Verification items for the finished model (mm, model axes). Face numbers are marked on the shaded views. A direction names the side the tool comes from. Round coordinates to 2 decimals unless told otherwise and drop trailing zeros. Order: outer loops, then holes, each group sorted by start corner. A loop starts at its lowest first (then second) coordinate and runs counter-clockwise, first axis right, second up. Notation, with made-up numbers: (-37.75, 41.5) -> (6.25, 41.5) arc R12 ccw to (6.25, 46.5) -> close; hole circle Ø6 at (-17, 21.25). An arc over 180 degrees is marked (long way). Return JSON: item names as keys, results as strings. Group by question number.
Item 1: Access from +Z, -Z, +X, -X, +Y, -Y to the whole of each face (thin tool, end or side, straight path). Record for the marked faces 1, 2 and 3.
Item 2: Sectioned sample at D-D on z = 1.75. Record the cut outline in (x, y).
Item 3: Sectioned sample at B-B on x = 5. Record the cut outline in (y, z), plus the area to 3 significant figures.
Item 4: Sectioned sample at A-A on y = -10. Record the cut outline in (x, z), plus the area to 3 significant figures.
Item 5: Sectioned sample at C-C on x = 1.25. Record the cut outline in (y, z), plus the area to 3 significant figures.
Item 6: Scan lines: probe 1 along Y at (x, z) = (5, -8.95); probe 2 along Y at (x, z) = (5, 1.6); probe 3 along Y at (x, z) = (4.25, -2). Record each from-to range of solid material in increasing order. Write a range as from..to.
Item 7: Depth check by flat-ended pin: pin 1 Ø3.5 at (x, y) = (5, -10) entering from +Z; pin 2 Ø3 at (x, z) = (7, -3.5) entering from -Y; pin 3 Ø3 at (x, z) = (3, -5) entering from +Y. Enter the tip coordinate at first touch or a pass-through.
Item 8: Draft check along Y on the marked faces 4, 5, 6 and 7. Enter one of: pulls with the +Y half, pulls with the -Y half, needs draft (parallel to the pull), parting line crosses it, or undercut.
```python
from build123d import *

# Parameters (mm, degrees)
SKETCH1_W           = 10
SKETCH1_H           = 15
SKETCH1_R           = 3
SKETCH1_H_2         = 3
BOSS_EXTRUDE1_DEPTH = 3
SKETCH1_4_W         = 10
SKETCH1_4_H         = 3
BOSS_EXTRUDE2_DEPTH = 10
BOSS_EXTRUDE3_START = -10
SKETCH1_5_W         = 10
SKETCH1_5_H         = 10
SKETCH1_5_R         = 3
BOSS_EXTRUDE3_DEPTH = 3


with BuildPart() as part:
    # Sketch1 → Boss-Extrude1 (new body)
    # profile 1 of 2: a face of its own
    with BuildSketch(Plane.XY):
        with Locations((5, -7.5)):
            Rectangle(SKETCH1_W, SKETCH1_H)
        with Locations((5, -10)):
            Circle(SKETCH1_R, mode=Mode.SUBTRACT)
    # profile 2 of 2: a face of its own
    with BuildSketch(Plane.XY):
        with Locations((5, 1.5)):
            Rectangle(SKETCH1_W, SKETCH1_H_2)
    extrude(amount=BOSS_EXTRUDE1_DEPTH)

    # Sketch1<4> → Boss-Extrude2 (add)
    with BuildSketch(Plane.XY):
        with Locations((5, 1.5)):
            Rectangle(SKETCH1_4_W, SKETCH1_4_H)
    extrude(amount=-BOSS_EXTRUDE2_DEPTH)

    # Sketch1<5> → Boss-Extrude3 (add)
    with BuildSketch(Plane.XY.offset(BOSS_EXTRUDE3_START)):
        with Locations((5, 8)):
            Rectangle(SKETCH1_5_W, SKETCH1_5_H)
        with Locations((5, 8)):
            Circle(SKETCH1_5_R, mode=Mode.SUBTRACT)
    extrude(amount=BOSS_EXTRUDE3_DEPTH)


solid = part.part
```
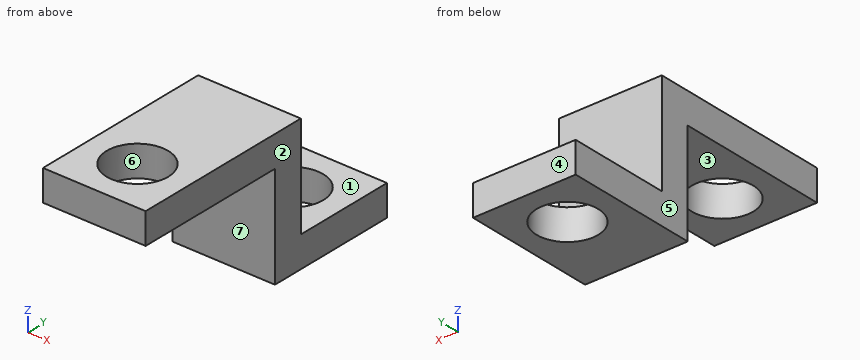
Recorded:
{
 "1": {"face 1": "+Z, +X, -X, +Y", "face 2": "+Z, -Z, +X, +Y, -Y", "face 3": "-Z, +X, -X, -Y"},
 "2": {"outline": "(0, -15) -> (10, -15) -> (10, 3) -> (0, 3) -> close; hole circle Ø6 at (5, -10)"},
 "3": {"outline": "(-15, 0) -> (-13, 0) -> (-13, 3) -> (-15, 3) -> close; (-7, 0) -> (0, 0) -> (0, -10) -> (5, -10) -> (5, -7) -> (3, -7) -> (3, 3) -> (-7, 3) -> close; (11, -10) -> (13, -10) -> (13, -7) -> (11, -7) -> close", "area": "78.0 mm²"},
 "4": {"outline": "(0, 0) -> (2, 0) -> (2, 3) -> (0, 3) -> close; (8, 0) -> (10, 0) -> (10, 3) -> (8, 3) -> close", "area": "12.0 mm²"},
 "5": {"outline": "(-15, 0) -> (0, 0) -> (0, -10) -> (13, -10) -> (13, -7) -> (3, -7) -> (3, 3) -> (-15, 3) -> close", "area": "114 mm²"},
 "6": {"probe 1": "0..5, 11..13", "probe 2": "-15..-13, -7..3", "probe 3": "0..3"},
 "7": {"pin 1": "through", "pin 2": "y = 0", "pin 3": "y = 3"},
 "8": {"face 4": "pulls with the +Y half", "face 5": "needs draft", "face 6": "undercut", "face 7": "pulls with the -Y half"}
}
